Verification items for the finished model (mm, model axes). Coordinates: 2 decimals unless noted, no trailing zeros. Answer in a Markdown table with one row per item.
Autodesk Inventor part; units mm, degrees
ref_plane "YZ Plane" through (0, 0, 0) normal (1, 0, 0) x (0, 1, 0)
ref_plane "XZ Plane" through (0, 0, 0) normal (0, 1, 0) x (-1, 0, 0)
ref_plane "XY Plane" through (0, 0, 0) normal (0, 0, 1) x (1, 0, 0)
sketch "Sketch1" plane through (0, 0, 0) normal (1, 0, 0) x (0, 1, 0)
  line L0 (2.1391, 3.4522) -> (-2.6609, 3.4522)
  line L1 (-2.6609, 3.4522) -> (-2.6609, -3.5478)
  line L2 (-2.6609, -3.5478) -> (2.1391, -3.5478)
  line L3 (2.1391, -3.5478) -> (2.1391, 3.4522)
  point P0 (0, 0)
  dimension "d0" = 4.8
  dimension "d1" = 7
extrude "Extrusion1" add sketch "Sketch1" along normal blind 200
sketch "Sketch2" plane through (0, 2.1391, 3.4522) normal (0, 1, 0) x (1, 0, 0)
  circle A0 centre (10, 3.5) radius 1.2
  line L0 (0, 7) -> (0, 0)
  line L1 (0, 0) -> (200, 0)
  circle A1 centre (30, 3.5) radius 1.2
  circle A2 centre (50, 3.5) radius 1.2
  circle A3 centre (70, 3.5) radius 1.2
  circle A4 centre (90, 3.5) radius 1.2
  circle A5 centre (110, 3.5) radius 1.2
  circle A6 centre (130, 3.5) radius 1.2
  circle A7 centre (150, 3.5) radius 1.2
  circle A8 centre (170, 3.5) radius 1.2
  circle A9 centre (190, 3.5) radius 1.2
  point P0 (0, 3.4522)
  dimension "d4" = 2.4
  dimension "d5" = 10
  dimension "d6" = 3.5
  dimension "d9" = 20
extrude "Extrusion2" cut sketch "Sketch2" against normal through all
properties part number "MGN7Cx200mm_rail"
1) Depth check by flat-ended pin: pin 1 (2 mm diameter, centred on x = 110, z = -0.05, fed in from +Y). Enter the tip coordinate at first touch or a pass-through.
Response values:
| item | result |
|---|---|
| pin 1 | passes through |
2) Thickness scan on L1, parallel to Z at x = 30, y = -0.25. Record the ranges inside material, lowest first. Write a range as [from, to].
Response values:
| item | result |
|---|---|
| L1 | z = [-3.55, -1.25], [1.15, 3.45] |
3) Sectioned sample at A-A (y = -1.15). Give the number of separate pieces and of enclosed holes in the cut face, then the cut area to 3 significant figures.
Response values:
| item | result |
|---|---|
| separate pieces | 1 |
| enclosed holes | 10 |
| area | 1,350 mm² |
